For this review, take the finished solid that the model builds, in its own axes (mm). A direction names the side the tool comes from. Give positions to 0.01 mm unless a question says otherwise; leave off trailing zeros. Order: outer loops, then holes, each group sorted by start corner. A loop starts at its lowest first (then second) coordinate and runs counter-clockwise, first axis right, second up. Notation, with made-up numbers: (-36.5, 27) -> (9.5, 27) arc R33 ccw to (9.5, 55) -> close; hole circle Ø7 at (72, 14). An arc over 180 degrees is marked (long way). Return JSON: item names as keys, results as strings. Group by question number.
1) Insertion check: P1, Ø4, axis at x = -38, y = 21.5, coming from the -Z side; P2, Ø1.7, axis at x = -30.5, z = 3, coming from the -Y side; P3, Ø1, axis at y = 8.5, z = 1.5, coming from the -X side; P4, Ø3, axis at x = -20, z = 4.5, coming from the +Y side. Each pin has a flat end and moves straight along its axis. Give the tip position at first contact, or say it passes through.
2) Add section D-D (x = -27.5). Give the boundary of the cut face in (y, z).
3) The part is to be moulded in two halves that separate along X. For faces 6 (the face through (-39.375, 20.785, 2.89)), 7 (the face through (5, 40, 3)), 8 (the face through (-27, 22, 4.25)), 9 (the face through (-3.01, 11.65, 2.81)), say which applies: released by +X, released by -X, zero draft, split by the parting line, or undercut.
4) Add section C-C (z = 1). Give the boundary of the cut face in (x, y), then the cut area to 3 significant figures.
5) Add section B-B (y = 21.5). Give the boundary of the cut face in (x, z).
6) Add section A-A (x = -38). Give the boundary of the cut face in (y, z), then the cut area to 3 significant figures.
7) To check wall thickness, follow line 1 along X through (y, z) = (21.5, 3.2); line 2 along Y through (x, z) = (27, 2.5); line 3 along Y through (x, z) = (-27.5, 2.75). State the ranges of each line that lie inside material, in increasing order.
8) For faces 1 (the face through (0, 41, 3)), 2 (the face through (-29, 20.1, 2.1)), 3 (the face through (24, 2, 3)), 4 (the face through (4, 22, 3)), 5 (the face through (0, 2, 3)), list the 3-axis set-ups (+Z, -Z, +X, -X, +Y, -Y) from which the entire face can be reached by the end or side of a thin tool; tool diameter is ignored.
Solid Edge part; units mm, degrees
sketch "Sketch1" plane through (0, 0, 0) normal (0, 0, 1) x (1, 0, 0)
  line L0 (4, 39) -> (4, 4)
  line L1 (4, 4) -> (43, 4)
  line L2 (43, 4) -> (43, 0)
  line L3 (0, 0) -> (43, 0)
  line L4 (0, 43) -> (0, 0)
  line L5 (43, 43) -> (0, 43)
  line L6 (43, 43) -> (43, 39)
  line L7 (43, 39) -> (4, 39)
extrude "Protrusion1" add sketch "Sketch1" along normal blind 5.7
sketch "Sketch2" plane through (43, 41, 2.85) normal (1, 0, 0) x (0, 1, 0)
  line L0 (-2, 0.85) -> (0, 0.85)
  line L1 (0, 0.85) -> (0, -0.85)
  line L2 (0, -0.85) -> (-2, -0.85)
  line L3 (-2, -0.85) -> (-2, 0.85)
  line L4 (-37, -0.85) -> (-37, 0.85)
  line L5 (-37, 0.85) -> (-39, 0.85)
  line L6 (-39, 0.85) -> (-39, -0.85)
  line L7 (-39, -0.85) -> (-37, -0.85)
extrude "VaciadoExtruido_1" cut sketch "Sketch2" against normal blind 38
sketch "Sketch3" plane through (21.5, 21.5, 5.7) normal (0, 0, 1) x (1, 0, 0)
  line L0 (-66.5, 7) -> (-21.5, 7)
  line L1 (-21.5, 7) -> (-21.5, -7)
  line L2 (-21.5, -7) -> (-66.5, -7)
  line L3 (-66.5, -7) -> (-66.5, 7)
extrude "VaciadoExtruido_2" add sketch "Sketch3" against normal blind 5.7
sketch "Sketch4" plane through (11, 21.5, 0) normal (0, 0, -1) x (1, 0, 0)
  circle A0 centre (-38.5, 0) radius 2.05
extrude "VaciadoExtruido_3" cut sketch "Sketch4" against normal blind 4.25
sketch "Sketch5" plane through (11, 21.5, 5.7) normal (0, 0, 1) x (0, -1, 0)
  circle A0 centre (0, -49) radius 1.55
extrude "Cutout1" cut sketch "Sketch5" against normal up to next
fillet "Redondeo_1" radius 10 2 edges at (0, 14.5, 2.85) (0, 28.5, 2.85)
Evaluation:
{
 "1": {"P1": "z = 0", "P2": "y = 14.5", "P3": "x = -1.07", "P4": "y = 28.5"},
 "2": {"outline": "(14.5, 0) -> (19.45, 0) -> (19.45, 4.25) -> (23.55, 4.25) -> (23.55, 0) -> (28.5, 0) -> (28.5, 5.7) -> (14.5, 5.7) -> close"},
 "3": {"face 6": "undercut", "face 7": "released by +X", "face 8": "undercut", "face 9": "released by -X"},
 "4": {"outline": "(-45, 14.5) -> (-10, 14.5) arc R10 cw to (0, 4.5) -> (0, 0) -> (43, 0) -> (43, 4) -> (4, 4) -> (4, 39) -> (43, 39) -> (43, 43) -> (0, 43) -> (0, 38.5) arc R10 cw to (-10, 28.5) -> (-45, 28.5) -> close; hole circle Ø3.1 at (-38, 21.5); hole circle Ø4.1 at (-27.5, 21.5)", "area": "1,140 mm^2"},
 "5": {"outline": "(-45, 0) -> (-39.55, 0) -> (-39.55, 5.7) -> (-45, 5.7) -> close; (-36.45, 0) -> (-29.55, 0) -> (-29.55, 4.25) -> (-25.45, 4.25) -> (-25.45, 0) -> (4, 0) -> (4, 5.7) -> (-36.45, 5.7) -> close"},
 "6": {"outline": "(14.5, 0) -> (19.95, 0) -> (19.95, 5.7) -> (14.5, 5.7) -> close; (23.05, 0) -> (28.5, 0) -> (28.5, 5.7) -> (23.05, 5.7) -> close", "area": "62.1 mm^2"},
 "7": {"line 1": "-45 to -39.55, -36.45 to -29.55, -25.45 to 4", "line 2": "0 to 2, 41 to 43", "line 3": "14.5 to 19.45, 23.55 to 28.5"},
 "8": {"face 1": "+Z, -Z, -X, +Y", "face 2": "-Z", "face 3": "+X", "face 4": "+Z, -Z, +X", "face 5": "+Z, -Z, -X, -Y"}
}
